Part print with two shaded views. Sizes in mm from the minimum x, y, z corner. A direction names the side the tool comes from. Give positions to 0.01 mm unless a question says otherwise; leave off trailing zeros. Write each loop counter-clockwise with the first axis right and the second up, starting at its lowest first coordinate (ties: lowest second). Pieces come first, ordered by that corner, then holes. Notation, with made-up numbers: (74.5, 88) - (98.5, 88) arc R28 ccw to (98.5, 122) - close; hole circle Ø2 at (71.5, 38.25). An arc over 180 degrees is marked (long way). One line per item, written item: value. Start each with the question number.
(1) Cut at D-D, the plane x = 509. List the corners of the cut face in (y, z), and give its area (3 significant figures).
(2) Cut at C-C, the plane y = 499. List the corners of the cut face in (x, z).
(3) Cut at B-B, the plane z = 150. List the corners of the cut face in (x, y), and give its area (3 significant figures).
(4) Cut at A-A, the plane x = 700. List the corners of the cut face in (y, z).
(5) Drop flat-ended pins along their axis: P1, Ø3, axis at x = 607, z = 495.5, coming from the +Y side; P2, Ø2, axis at y = 296.5, z = 1113, coming from the +X side; P3, Ø12, axis at x = 169.5, y = 531, coming from the -Z side. Give the stop position or say it passes through.
(6) Probe L1, parallel to Z at x = 787, y = 530; L2, parallel to Y at x = 45, z = 1001.5; L3, parallel to X at y = 396, z = 165.5. List the from-to ranges inside material, lowest first.
(7) 3-axis set-ups, long thin cutter, end or side, ignore diameter. For the marked faces 1 and 2: which of +Z, -Z, +X, -X, +Y, -Y reach the whole face in a straight line?
(8) Mould opens along Z. For the marked faces 3, 4, 5 and 6 say: pulls with the +Z half, pulls with the -Z half, needs draft (parallel to the pull), parting line crosses it, or undercut.
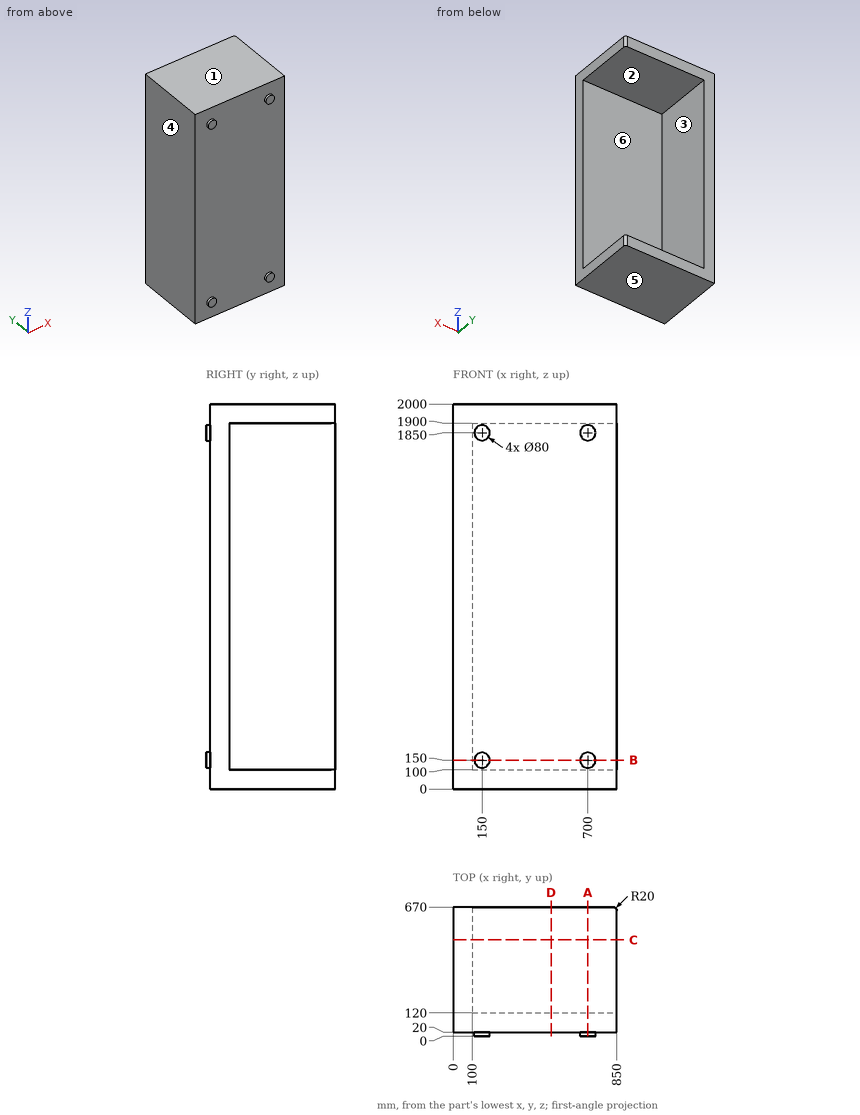
Answers follow:
1. outline: (20, 0) - (670, 0) - (670, 100) - (120, 100) - (120, 1900) - (670, 1900) - (670, 2000) - (20, 2000) - close
1. area: 310,000 mm²
2. outline: (0, 0) - (850, 0) - (850, 100) - (100, 100) - (100, 1900) - (850, 1900) - (850, 2000) - (0, 2000) - close
3. outline: (0, 20) - (110, 20) - (110, 0) - (190, 0) - (190, 20) - (660, 20) - (660, 0) - (740, 0) - (740, 20) - (850, 20) - (850, 120) - (100, 120) - (100, 670) - (0, 670) - close
3. area: 143,000 mm²
4. outline: (0, 110) - (20, 110) - (20, 0) - (670, 0) - (670, 100) - (120, 100) - (120, 1900) - (670, 1900) - (670, 2000) - (20, 2000) - (20, 1890) - (0, 1890) - (0, 1810) - (20, 1810) - (20, 190) - (0, 190) - close
5. P1: stops at y = 120
5. P2: stops at x = 100
5. P3: stops at z = 0
6. L1: z = 0 to 100, 1900 to 2000
6. L2: y = 20 to 670
6. L3: x = 0 to 100
7. face 1: +Z, +X, -X, +Y, -Y
7. face 2: +X, +Y
8. face 3: undercut
8. face 4: needs draft
8. face 5: pulls with the -Z half
8. face 6: undercut
